Autodesk Inventor part; units mm, degrees
ref_plane "YZ Plane" through (0, 0, 0) normal (1, 0, 0) x (0, 1, 0)
ref_plane "XZ Plane" through (0, 0, 0) normal (0, 1, 0) x (-1, 0, 0)
ref_plane "XY Plane" through (0, 0, 0) normal (0, 0, 1) x (1, 0, 0)
sketch "Sketch1" plane through (0, 0, 0) normal (0, 0, 1) x (1, 0, 0)
  circle A0 centre (0, 0) radius 4
  line L0 (1.1547, 2) -> (2.3094, 0)
  line L1 (2.3094, 0) -> (1.1547, -2)
  line L2 (1.1547, -2) -> (-1.1547, -2)
  line L3 (-1.1547, -2) -> (-2.3094, 0)
  line L4 (-2.3094, 0) -> (-1.1547, 2)
  line L5 (-1.1547, 2) -> (1.1547, 2)
  dimension "d0" = 8
  dimension "d1" = 4
extrude "Extrusion1" add sketch "Sketch1" against normal blind 2
sketch "Sketch2" plane through (0, 0, -2) normal (0, 0, -1) x (-1, 0, 0)
  circle A0 centre (0, 0) radius 4
extrude "Extrusion2" add sketch "Sketch2" along normal blind 1
sketch "Sketch3" plane through (0, 0, -3) normal (0, 0, -1) x (-1, 0, 0)
  circle A0 centre (0, 0) radius 2
  dimension "d6" = 4
extrude "Extrusion3" add sketch "Sketch3" along normal blind 8
fillet "Fillet1" radius 0.2 3 edges at (4, 0, -3) (-4, 0, 0) (2, 0, -11)
thread "Thread1"
properties part number "M3 x 8 Socket Head Bolt"
CAD build for the part. Positions are in the model's coordinates, mm. A direction names the side the tool comes from. Give positions to 0.01 mm unless a question says otherwise; leave off trailing zeros. Order: outer loops, then holes, each group sorted by start corner. A loop starts at its lowest first (then second) coordinate and runs counter-clockwise, first axis right, second up.
(1) Flat gauge pins, fed straight in: pin 1 (3 mm diameter, centred on y = -2.5, z = -6, fed in from -X); pin 2 (0.6 mm diameter, centred on x = 0.5, z = -0.5, fed in from -Y) (3 decimals); pin 3 (2 mm diameter, centred on x = 0, y = 0.5, fed in from +Z). Where does each tip first touch, or does it go through?
(2) Saw through at B-B, the plane z = -9.25. Give the cut face in (x, y), then the cut area to 3 significant figures.
(3) Mould opens along X. For faces 3 (the flat face through (0, -2, -1)), 4 (the cylindrical face through (0, 2, -7)), 5 (the flat face through (-2, -2, -3)) say: released by +X, released by -X, zero draft, split by the parting line, or undercut.
(4) Saw through at A-A, the plane x = 0. Give the cut face in (y, z), then the cut area to 3 significant figures.
(5) Drill centre lines: L1, parallel to Z at x = -1.75, y = -3; L2, parallel to Y at x = 0, z = -10; L3, parallel to Z at x = 1.5, y = -1. Where is each one in solid material? Low to high.
(6) Tool access for faces 1 (the flat face through (-1.74, 0.99, -0.99)), 2 (the flat face through (0, 0, -11)): list every direction of +Z, -Z, +X, -X, +Y, -Y with a clear straight run to the whole face (end or side of a thin tool).
Results found:
1. pin 1: stops at x = -1.73
1. pin 2: stops at y = -3.995
1. pin 3: stops at z = -2
2. outline: circle Ø4 at (0, 0)
2. area: 12.6 mm2
3. face 3: undercut
3. face 4: split by the parting line
3. face 5: zero draft
4. outline: (-4, -2.8) arc R0.2 ccw to (-3.8, -3) - (-2, -3) - (-2, -10.8) arc R0.2 ccw to (-1.8, -11) - (1.8, -11) arc R0.2 ccw to (2, -10.8) - (2, -3) - (3.8, -3) arc R0.2 ccw to (4, -2.8) - (4, -0.2) arc R0.2 ccw to (3.8, 0) - (2, 0) - (2, -2) - (-2, -2) - (-2, 0) - (-3.8, 0) arc R0.2 ccw to (-4, -0.2) - close
4. area: 47.9 mm2
5. L1: z = -3 to 0
5. L2: y = -2 to 2
5. L3: z = -11 to -2
6. face 1: +Z
6. face 2: -Z, +X, -X, +Y, -Y
